from build123d import *

# Parameters (mm, degrees)
F1_DEPTH = 35
F3_W     = 14.1933254312
F3_H     = 10
F4_DEPTH = 5
F6_DEPTH = 5
F8_DEPTH = 0.5
F9_DEPTH = 200


with BuildPart() as f1:
    # F0 (on Right) → F1 (new body, symmetric)
    with BuildSketch(Plane.YZ):
        Polygon((4.0779394949, -1.9816074769), (-5.5346774645, 0.7747660812), (-3.7443463919, 7.0183925231), (-6.5346774645, 7.0183925231), (-6.5346774645, -2.9816074769), (7.6586479667, -2.9816074769), (7.6586479667, 7.0183925231), (6.6586479667, 7.0183925231), align=None)
    extrude(amount=F1_DEPTH, both=True)


with BuildPart() as f1_1:
    # F2: moved
    add(f1.part.moved(Location((0, 0, 2.9817))))

    # F3 (on face) → F4 (join)
    with BuildSketch(Plane(origin=(-35, 0, 0), x_dir=(0, -1, 0), z_dir=(-1, 0, 0))):
        with Locations((-0.5619852511, 5.0000925231)):
            Rectangle(F3_W, F3_H)
    extrude(amount=F4_DEPTH)

    # F5 (on face) → F6 (join)
    with BuildSketch(Plane.YZ.offset(35)):
        Polygon((-3.7443463919, 10.0000925231), (-6.5346774645, 10.0000925231), (-6.5346774645, 9.25231e-05), (7.6586479667, 9.25231e-05), (7.6586479667, 10.0000925231), (6.6586479667, 10.0000925231), (4.0779394949, 1.0000925231), (-5.5346774645, 3.7564660812), align=None)
        Polygon((6.6586479667, 10.0000925231), (-3.7443463919, 10.0000925231), (-5.5346774645, 3.7564660812), (4.0779394949, 1.0000925231), align=None)
    extrude(amount=F6_DEPTH)

    # F8 (add): a face of the model
    f8_faces = [f1_1.faces().sort_by_distance(p)[0] for p in [
        (0, -6.5346774645, 5.0000925231),
    ]]
    extrude(f8_faces, amount=F8_DEPTH)

    # F7 (on face) → F9 (cut)
    with BuildSketch(Plane(origin=(0, 0.574809482, 2.00459889), x_dir=(1, 0, 0), z_dir=(0, 0.2756373558, 0.9612616959))):
        Polygon((15, 3.6443041761), (0, 3.6443041761), (-15, 3.6443041761), (-15, -6.3556958239), (15, -6.3556958239), align=None)
    extrude(amount=-F9_DEPTH, mode=Mode.SUBTRACT)


solid = f1_1.part
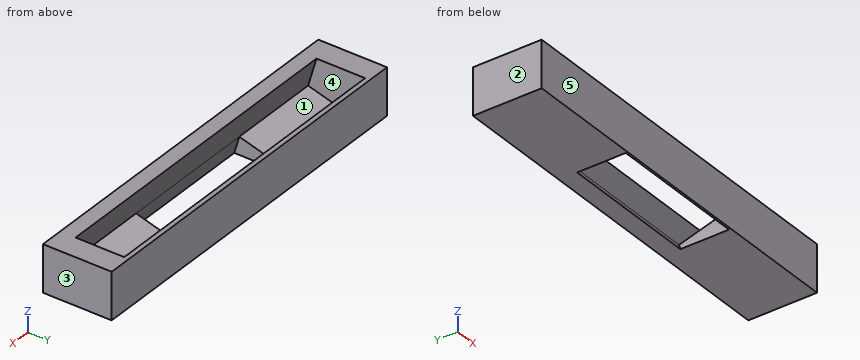
Geometry: final body of the model. Coordinates: model frame, mm. Face numbers are marked on the shaded views. A direction names the side the tool comes from. Give positions to 0.01 mm unless a question says otherwise; leave off trailing zeros. Loops run counter-clockwise (first coordinate to the right, second up) from the corner with the lowest first, then second, coordinate; pieces in that order, holes last. Notation, with made-up numbers: M 42.5,54 L 78.5,54 A14 cw 78.5,77 Z; hole C 21,-22.75 d3. An arc over 180 degrees is marked long. Put each result on its own line as item: value. Start each with the question number.
1) Cut plane D-D (x = -18). Output: boundary loops of the cut face in (y, z).
2) Cut plane B-B (y = -1.75). Output: boundary loops of the cut face in (x, z).
3) Ray query, line 1 along X through (y, z) = (-1.75, 8.5); line 2 along Y through (x, z) = (-3.5, 5.5); line 3 along X through (y, z) = (-6, 1.75). Return the intervals inside material, ascending.
4) Cut plane A-A (x = 6). Output: boundary loops of the cut face in (y, z), then the cut area to 3 significant figures.
5) Access query for the marked faces 1 and 2. Directions: +Z, -Z, +X, -X, +Y, -Y. A direction counts if a zero-diameter tool reaches every point of the face in a straight line with its end or side. Return the directions, or none.
6) Cut plane C-C (z = 3). Output: boundary loops of the cut face in (x, y), then the cut area to 3 significant figures.
7) Pull-direction query (X, two-part tool) for the marked faces 3, 4 and 5; classes: pulls with the +X half, pulls with the -X half, needs draft (parallel to the pull), parting line crosses it, or undercut.
Verdict:
1. outline: M -7.03,0 L 7.66,0 L 7.66,10 L 6.66,10 L 4.08,1 L -5.53,3.76 L -3.74,10 L -7.03,10 Z
2. outline: M -40,0 L -15,0 L -15,2.67 L -35,2.67 L -35,10 L -40,10 Z; M 15,0 L 40,0 L 40,10 L 35,10 L 35,2.67 L 15,2.67 Z
3. line 1: -40 to -35, 35 to 40
3. line 2: -7.03 to -5.03, 5.37 to 7.66
3. line 3: -40 to -15, 15 to 40
4. outline: M -7.03,0 L -6.61,0 L -3.74,10 L -7.03,10 Z; M 3.79,0 L 7.66,0 L 7.66,10 L 6.66,10 Z
4. area: 42.9 mm2
5. face 1: none
5. face 2: +Z, -Z, -X, +Y, -Y
6. outline: M -40,-7.03 L 40,-7.03 L 40,7.66 L -40,7.66 Z; hole M -35,-2.9 L -15,-2.9 L -15,-5.75 L 15,-5.75 L 15,-2.9 L 35,-2.9 L 35,4.65 L -35,4.65 Z
6. area: 561 mm2
7. face 3: pulls with the +X half
7. face 4: undercut
7. face 5: needs draft
